Can you work these out from the drawing? Everything is in mm from the part's minimum corner. A direction names the side the tool comes from. Round coordinates to 2 decimals unless told otherwise and drop trailing zeros. Order: outer loops, then holes, each group sorted by start corner. A loop starts at its lowest first (then second) coordinate and runs counter-clockwise, first axis right, second up. Notation, with made-up numbers: (49.5, 26.25) -> (103.5, 26.25) arc R11 cw to (103.5, 43.25) -> close; hole circle Ø8 at (-11, 73). An arc over 180 degrees is marked (long way). One line per item, written item: value.
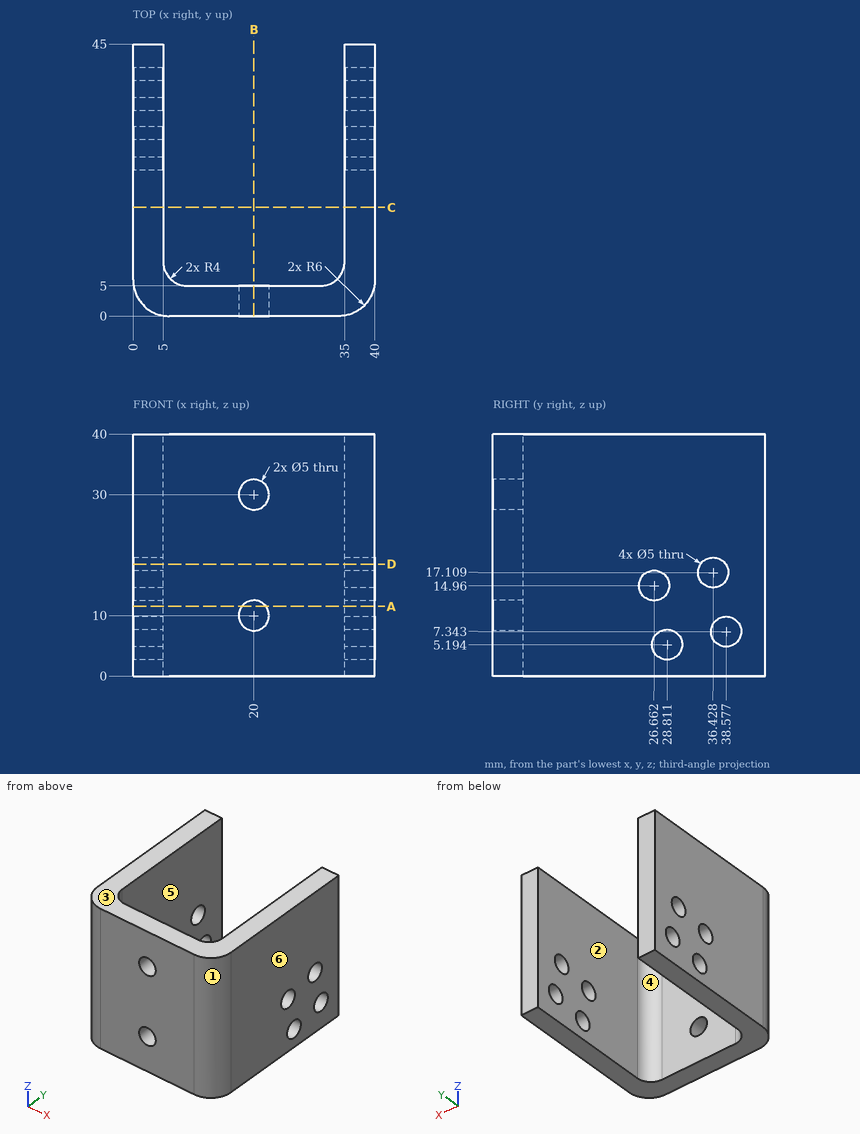
Q1. I want a section at A-A on z = 11.5. List the corners of the cut face in (x, y) for me.
Answers below:
outline: (0, 6) arc R6 ccw to (6, 0) -> (18, 0) -> (18, 5) -> (9, 5) arc R4 cw to (5, 9) -> (5, 45) -> (0, 45) -> close; (22, 0) -> (34, 0) arc R6 ccw to (40, 6) -> (40, 45) -> (35, 45) -> (35, 9) arc R4 cw to (31, 5) -> (22, 5) -> close
Q2. I want a section at B-B on x = 20. List the corners of the cut face in (y, z) for me, plus the area to 3 significant figures.
Answers below:
outline: (0, 0) -> (5, 0) -> (5, 7.5) -> (0, 7.5) -> close; (0, 12.5) -> (5, 12.5) -> (5, 27.5) -> (0, 27.5) -> close; (0, 32.5) -> (5, 32.5) -> (5, 40) -> (0, 40) -> close
area: 150 mm^2
Q3. Please list where these lines run through material, in increasing order: line 1 along X through (y, z) = (21.5, 32.5); line 2 along Z through (x, y) = (20, 2); line 3 along Y through (x, z) = (13.5, 33.5).
Answers below:
line 1: 0 to 5, 35 to 40
line 2: 0 to 7.5, 12.5 to 27.5, 32.5 to 40
line 3: 0 to 5
Q4. We'd pull the mould along X, two halves only. Please class the marked faces 3, 4, 5 and 6: released by +X, released by -X, zero draft, split by the parting line, or undercut.
Answers below:
face 3: zero draft
face 4: undercut
face 5: undercut
face 6: released by +X
Q5. I want a section at D-D on z = 18.5. Give the number of separate pieces and of enclosed holes in the cut face, plus the area to 3 significant figures.
Answers below:
separate pieces: 3
enclosed holes: 0
area: 550 mm^2
Q6. I want a section at C-C on y = 18. List the corners of the cut face in (x, z) for me, plus the area to 3 significant figures.
Answers below:
outline: (0, 0) -> (5, 0) -> (5, 40) -> (0, 40) -> close; (35, 0) -> (40, 0) -> (40, 40) -> (35, 40) -> close
area: 400 mm^2
Q7. Will these pins go through, and if not, where does the flat tip stop? pin 1 Ø11 at (x, z) = (25, 14) entering from +Y; pin 2 Ø4.5 at (y, z) = (26.66, 14.96) entering from +X.
Answers below:
pin 1: y = 5
pin 2: through
Q8. On a 3-axis mill with a long thin cutter (end or side, diameter ignored), from which of +Z, -Z, +X, -X, +Y, -Y can I reach the whole of each face in a straight line? I mean the marked faces 1 and 2. Say none if no direction works.
Answers below:
face 1: +Z, -Z, +X, -Y
face 2: +Z, -Z, +Y
